from build123d import *

# Parameters (mm, degrees)
SKETCH_R          = 6
SKETCH_R_2        = 3
SKETCH_R_3        = 0.25
PAD_DEPTH         = 12
CYLINDER_R        = 6
CYLINDER_DEPTH    = 8
CYLINDER001_R     = 4.5
CYLINDER001_DEPTH = 8
CYLINDER002_R     = 4.5
CYLINDER002_DEPTH = 4
CYLINDER003_R     = 4
CYLINDER003_DEPTH = 4
CYLINDER004_R     = 3.5
CYLINDER004_DEPTH = 8


with BuildPart() as part:
    # Sketch → Pad (new body)
    with BuildSketch(Plane.XY):
        Circle(SKETCH_R)
        Circle(SKETCH_R_2, mode=Mode.SUBTRACT)
        with Locations((-5, 0)):
            Circle(SKETCH_R_3, mode=Mode.SUBTRACT)
        with Locations((5, 0)):
            Circle(SKETCH_R_3, mode=Mode.SUBTRACT)
        with Locations((0, 5)):
            Circle(SKETCH_R_3, mode=Mode.SUBTRACT)
        with Locations((0, -5)):
            Circle(SKETCH_R_3, mode=Mode.SUBTRACT)
    extrude(amount=PAD_DEPTH)

    # Cylinder → Cylinder (cut)
    with BuildSketch(Plane.XY):
        Circle(CYLINDER_R)
    extrude(amount=CYLINDER_DEPTH, mode=Mode.SUBTRACT)

    # Cylinder001 → Cylinder001 (join)
    with BuildSketch(Plane.XY):
        Circle(CYLINDER001_R)
    extrude(amount=CYLINDER001_DEPTH)

    # Cylinder002 → Cylinder002 (cut)
    with BuildSketch(Plane.XY):
        Circle(CYLINDER002_R)
    extrude(amount=CYLINDER002_DEPTH, mode=Mode.SUBTRACT)

    # Cylinder003 → Cylinder003 (join)
    with BuildSketch(Plane.XY):
        Circle(CYLINDER003_R)
    extrude(amount=CYLINDER003_DEPTH)

    # Cylinder004 → Cylinder004 (cut)
    with BuildSketch(Plane.XY):
        Circle(CYLINDER004_R)
    extrude(amount=CYLINDER004_DEPTH, mode=Mode.SUBTRACT)


solid = part.part
Could you check a few things on this model? Use its own coordinates, in mm. A direction names the side the tool comes from. Coordinates: 2 decimals unless noted, no trailing zeros. Write each loop counter-clockwise with the first axis right and the second up, starting at its lowest first coordinate (ties: lowest second). Pieces come first, ordered by that corner, then holes. Notation, with made-up numbers: (23.5, 12) - (50.5, 12) arc R18 cw to (50.5, 32) - close; hole circle Ø7 at (42.25, -13). An arc over 180 degrees is marked (long way). Put each result on its own line as item: value. Start each with the question number.
Q1. I want a section at D-D on z = 9.25. Write out the boundary of the cut face in (x, y), plus the area to 3 significant figures.
Q2. Which directions (+Z, -Z, +X, -X, +Y, -Y) give clear straight access to the entire face, cutting with the end or side of a thin tool? Please do faces 4 (the cylindrical face through (-6, 0, 10)), 5 (the flat face through (3, 1, 8)).
Q3. I want a section at A-A on y = 0. Write out the boundary of the cut face in (x, z).
Q4. I want a section at C-C on y = 2.5. Write out the boundary of the cut face in (x, z).
Q5. Please list where these lines run through material, in increasing order: L1, parallel to Y at x = 0, z = 10.95; L2, parallel to Z at x = -5, y = -3; L3, parallel to X at y = -5, z = 10.5.
Q6. Thinking about a two-plate mould opening in X: for faces 1 (the cylindrical face through (-0.867, -3.905, 1.972)), 2 (the flat face through (-3, -1, 12)), 3 (the cylindrical face through (3.233, -1.341, 3.944)), which applies, pulls with the +X half, pulls with the -X half, needs draft (parallel to the pull), parting line crosses it, or undercut?
Q7. I'm going to push flat-ended pins straight in: P1, Ø1.5, axis at y = 4.5, z = 8.5, coming from the +X side; P2, Ø2.5, axis at x = 1.5, y = -1.5, coming from the -Z side; P3, Ø1.5, axis at x = -4, z = 9.5, coming from the +Y side. Where does each tip first touch, or does it pass through?
Checks:
1. outline: circle Ø12 at (0, 0); hole circle Ø0.5 at (-5, 0); hole circle Ø6 at (0, 0); hole circle Ø0.5 at (0, -5); hole circle Ø0.5 at (0, 5); hole circle Ø0.5 at (5, 0)
1. area: 84.0 mm²
2. face 4: +Z, -Z
2. face 5: -Z
3. outline: (-6, 8) - (-5.25, 8) - (-5.25, 12) - (-6, 12) - close; (-4.75, 8) - (-4.5, 8) - (-4.5, 4) - (-4, 4) - (-4, 0) - (-3.5, 0) - (-3.5, 8) - (-3, 8) - (-3, 12) - (-4.75, 12) - close; (3, 8) - (3.5, 8) - (3.5, 0) - (4, 0) - (4, 4) - (4.5, 4) - (4.5, 8) - (4.75, 8) - (4.75, 12) - (3, 12) - close; (5.25, 8) - (6, 8) - (6, 12) - (5.25, 12) - close
4. outline: (-5.45, 8) - (-3.74, 8) - (-3.74, 4) - (-3.12, 4) - (-3.12, 0) - (-2.45, 0) - (-2.45, 8) - (-1.66, 8) - (-1.66, 12) - (-5.45, 12) - close; (1.66, 8) - (2.45, 8) - (2.45, 0) - (3.12, 0) - (3.12, 4) - (3.74, 4) - (3.74, 8) - (5.45, 8) - (5.45, 12) - (1.66, 12) - close
5. L1: -6 to -5.25, -4.75 to -3, 3 to 4.75, 5.25 to 6
5. L2: 8 to 12
5. L3: -3.32 to -0.25, 0.25 to 3.32
6. face 1: parting line crosses it
6. face 2: needs draft
6. face 3: undercut
7. P1: x = 4.68
7. P2: z = 8
7. P3: y = 5.04
